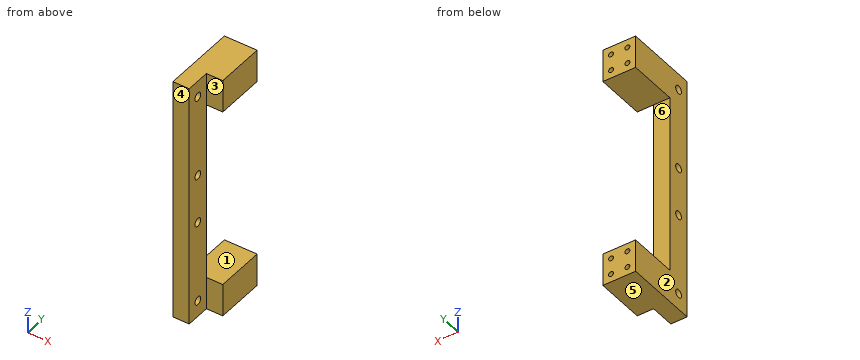
from build123d import *

# Parameters (mm, degrees)
SKETCH_1_W          = 10
SKETCH_1_H          = 150
EXTRUDE_1_DEPTH     = 15
SKETCH_2_W          = 20
SKETCH_2_H          = 20
EXTRUDE_2_DEPTH     = 30
SKETCH_3_R          = 2.5
CUT_EXTRUDE_1_DEPTH = 90.721792225
SKETCH_4_R          = 1.5
CUT_EXTRUDE_2_DEPTH = 10


with BuildPart() as part:
    # 草图1 → 凸台-拉伸1 (new body)
    with BuildSketch(Plane(origin=(0, 0, 0), x_dir=(1, 0, 0), z_dir=(0, 1, 0))):
        Rectangle(SKETCH_1_W, SKETCH_1_H)
    extrude(amount=EXTRUDE_1_DEPTH)

    # 草图2 → 凸台-拉伸2 (add)
    with BuildSketch(Plane(origin=(0, 15, 0), x_dir=(1, 0, 0), z_dir=(0, 1, 0))):
        with Locations((5, 65)):
            Rectangle(SKETCH_2_W, SKETCH_2_H)
        with Locations((5, -65)):
            Rectangle(SKETCH_2_W, SKETCH_2_H)
    extrude(amount=EXTRUDE_2_DEPTH)

    # 草图3 → 切除-拉伸1 (cut, through all)
    with BuildSketch(Plane.ZY.offset(5)):
        with Locations((-65, 7.5)):
            Circle(SKETCH_3_R)
        with Locations((-15, 7.5)):
            Circle(SKETCH_3_R)
        with Locations((15, 7.5)):
            Circle(SKETCH_3_R)
        with Locations((65, 7.5)):
            Circle(SKETCH_3_R)
    extrude(amount=-CUT_EXTRUDE_1_DEPTH, mode=Mode.SUBTRACT)

    # 草图4 → 切除-拉伸2 (cut)
    with BuildSketch(Plane(origin=(0, 45, 0), x_dir=(1, 0, 0), z_dir=(0, 1, 0))):
        with Locations(Location((0, 70, 0), (0, 0, 270))):
            Circle(SKETCH_4_R)
        with Locations(Location((10, 70, 0), (0, 0, 270))):
            Circle(SKETCH_4_R)
        with Locations(Location((0, 60, 0), (0, 0, 270))):
            Circle(SKETCH_4_R)
        with Locations(Location((10, 60, 0), (0, 0, 270))):
            Circle(SKETCH_4_R)
    cut_extrude_2 = extrude(amount=-CUT_EXTRUDE_2_DEPTH, mode=Mode.SUBTRACT)

    # 镜向1: 切除-拉伸2 across plane
    add(cut_extrude_2.mirror(Plane.XY), mode=Mode.SUBTRACT)


solid = part.part
Geometry check sheet. Reference: the model listing, model coordinates, mm. Face numbers are marked on the shaded views. A direction names the side the tool comes from. Give positions to 0.01 mm unless a question says otherwise; leave off trailing zeros. Order: outer loops, then holes, each group sorted by start corner. A loop starts at its lowest first (then second) coordinate and runs counter-clockwise, first axis right, second up.
1) Cross-section at A-A (z = -65). Record the boundary of the cut face in (x, y), then the cut area to 3 significant figures.
Results are:
outline: (-5, 0) - (5, 0) - (5, 5) - (-5, 5) - close; (-5, 10) - (5, 10) - (5, 15) - (15, 15) - (15, 45) - (-5, 45) - close
area: 700 mm2
2) Cross-section at D-D (z = 56.5). Record the boundary of the cut face in (x, y).
Results are:
outline: (-5, 0) - (5, 0) - (5, 15) - (15, 15) - (15, 45) - (-5, 45) - close
3) Material ranges on probe 1 along X at (y, z) = (39, 60); probe 2 along Z at (x, y) = (7.75, 34); probe 3 along X at (y, z) = (40, -59.5), recorded low to high.
Results are:
probe 1: x = -5 to -1.5, 1.5 to 8.5, 11.5 to 15
probe 2: z = -75 to -55, 55 to 75
probe 3: x = -5 to -1.41, 1.41 to 8.59, 11.41 to 15
4) Tool access check on the marked faces 1, 2 and 3. Record the directions out of +Z, -Z, +X, -X, +Y, -Y that give a thin tool (end or side, any length) a straight path to the whole face; none if there is none.
Results are:
face 1: +X, -X, +Y
face 2: +Z, -Z, -X, +Y, -Y
face 3: +Z, -Z, +X, -Y
5) Gauge pin test, flat ends, axial feed: pin 1 (1.5 mm diameter, centred on x = 0, z = -60, fed in from +Y); pin 2 (3.5 mm diameter, centred on x = 10, z = 69.5, fed in from +Y); pin 3 (5 mm diameter, centred on x = 10, z = -60, fed in from -Y); pin 4 (6 mm diameter, centred on y = 7.5, z = -65, fed in from +X). Record the tip position at first contact, or that the pin passes through.
Results are:
pin 1: stops at y = 35
pin 2: stops at y = 45
pin 3: stops at y = 15
pin 4: stops at x = 5
6) Cross-section at B-B (y = 24). Record the boundary of the cut face in (x, z), then the cut area to 3 significant figures.
Results are:
outline: (-5, -75) - (15, -75) - (15, -55) - (-5, -55) - close; (-5, 55) - (15, 55) - (15, 75) - (-5, 75) - close
area: 800 mm2
7) Cross-section at C-C (x = 0). Record the boundary of the cut face in (y, z).
Results are:
outline: (0, -75) - (45, -75) - (45, -71.5) - (35, -71.5) - (35, -68.5) - (45, -68.5) - (45, -61.5) - (35, -61.5) - (35, -58.5) - (45, -58.5) - (45, -55) - (15, -55) - (15, 55) - (45, 55) - (45, 58.5) - (35, 58.5) - (35, 61.5) - (45, 61.5) - (45, 68.5) - (35, 68.5) - (35, 71.5) - (45, 71.5) - (45, 75) - (0, 75) - close; hole circle Ø5 at (7.5, -65); hole circle Ø5 at (7.5, -15); hole circle Ø5 at (7.5, 15); hole circle Ø5 at (7.5, 65)
8) Draft check along Z on the marked faces 4, 5 and 6. Enter one of: released by +Z, released by -Z, zero draft, split by the parting line, or undercut.
Results are:
face 4: zero draft
face 5: released by -Z
face 6: undercut
